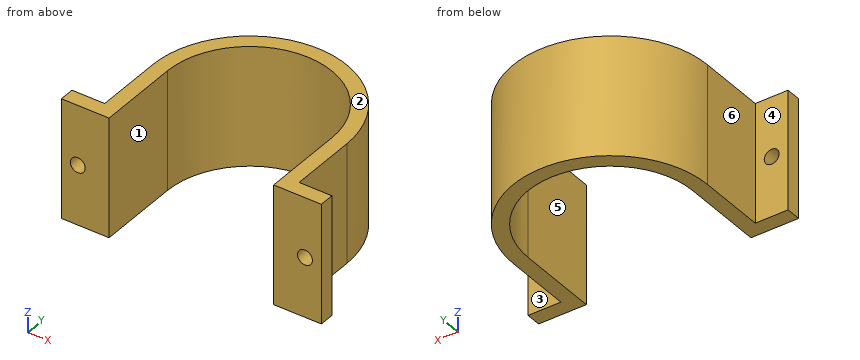
Autodesk Inventor part; units mm, degrees
ref_plane "YZ Plane" through (0, 0, 0) normal (1, 0, 0) x (0, 1, 0)
ref_plane "XZ Plane" through (0, 0, 0) normal (0, 1, 0) x (-1, 0, 0)
ref_plane "XY Plane" through (0, 0, 0) normal (0, 0, 1) x (1, 0, 0)
sketch "Sketch1" plane through (0, 0, 0) normal (0, 0, 1) x (1, 0, 0)
  arc A0 (17.526, 0) -> (-17.526, 0) centre (0, 0) ccw
  arc A1 (20.701, 0) -> (-20.701, 0) centre (0, 0) ccw
  line L0 (17.526, 0) -> (20.701, 0)
  line L1 (20.701, 0) -> (20.701, -17.526)
  line L2 (20.701, -17.526) -> (17.526, -17.526)
  line L3 (17.526, -17.526) -> (17.526, 0)
  line L4 (-20.701, 0) -> (-17.526, 0)
  line L5 (-17.526, 0) -> (-17.526, -17.526)
  line L6 (-17.526, -17.526) -> (-20.701, -17.526)
  line L7 (-20.701, -17.526) -> (-20.701, 0)
  line L8 (-17.526, -17.526) -> (-27.686, -17.526)
  line L9 (-27.686, -17.526) -> (-27.686, -14.351)
  line L10 (-27.686, -14.351) -> (-17.526, -14.351)
  line L11 (-17.526, -14.351) -> (-17.526, -17.526)
  line L12 (17.526, -17.526) -> (27.686, -17.526)
  line L13 (27.686, -17.526) -> (27.686, -14.351)
  line L14 (27.686, -14.351) -> (17.526, -14.351)
  line L15 (17.526, -14.351) -> (17.526, -17.526)
  point P0 (-20.701, -14.351)
  point P1 (20.701, -14.351)
  dimension "d0" = 17.526
  dimension "d1" = 3.175
  dimension "d23" = 3.175
  dimension "d24" = 17.526
  dimension "d25" = 3.175
  dimension "d26" = 17.526
  dimension "d27" = 10.16
  dimension "d28" = 3.175
  dimension "d29" = 10.16
  dimension "d30" = 3.175
extrude "Extrusion1" add sketch "Sketch1" along normal blind 25.4
sketch "Sketch5" plane through (-27.686, -14.351, 0) normal (0, 1, 0) x (1, 0, 0)
  line L0 (6.985, 0) -> (0, 0) construction
  line L1 (6.985, -25.4) -> (0, -25.4) construction
  line L2 (0, 0) -> (6.985, -25.4) construction
  line L3 (0, 0) -> (0, -25.4) construction
  line L4 (6.985, 0) -> (0, -25.4) construction
  line L5 (45.212, -25.4) -> (55.372, -25.4) construction
  line L6 (48.387, 0) -> (55.372, -25.4) construction
  line L7 (45.212, 0) -> (55.372, 0) construction
  line L8 (55.372, 0) -> (48.387, -25.4) construction
  point P0 (27.686, 0)
  point P1 (3.4925, -12.7)
sketch "Sketch6" plane through (20.701, -14.351, 0) normal (0, 1, 0) x (1, 0, 0)
  point P0 (-20.701, 0)
  point P1 (3.4926, -12.7006)
hole "Hole3" at (24.1936, -14.351, 12.7006) direction (0, -1, 0) diameter 3.175 end through all
hole "Hole4" at (-24.1935, -14.351, 12.7) direction (0, -1, 0) diameter 3.175 end through all
properties part number "ShootingMech_MotorMount"
Could you check a few things on this model? Use its own coordinates, in mm. Face numbers are marked on the shaded views. A direction names the side the tool comes from. Give positions to 0.01 mm unless a question says otherwise; leave off trailing zeros. Order: outer loops, then holes, each group sorted by start corner. A loop starts at its lowest first (then second) coordinate and runs counter-clockwise, first axis right, second up.
1. For pin 1 (3 mm diameter, centred on y = -12, z = 11, fed in from +X); pin 2 (3.5 mm diameter, centred on x = 25, z = 15.5, fed in from +Y); pin 3 (4 mm diameter, centred on x = -6, z = 5, fed in from +Y), each with a flat end and sliding along its axis, tell me the tip position at first contact or that it passes through.
Answers below:
pin 1: stops at x = 20.7
pin 2: stops at y = -14.35
pin 3: stops at y = 20.31
2. Which directions (+Z, -Z, +X, -X, +Y, -Y) give clear straight access to the entire face, cutting with the end or side of a thin tool? Please do the marked faces 1, 2 and 3.
Answers below:
face 1: +Z, -Z, -Y
face 2: +Z, +X, -X, +Y, -Y
face 3: +Z, -Z, +X, +Y
3. I need wall thicknesses on L1, parallel to X at y = -5, z = 3.5; L2, parallel to X at y = -15.7, z = 12.7; L3, parallel to X at y = 12, z = 6.5. Which ranges of each line are inside material? Lowest first, please.
Answers below:
L1: x = -20.7 to -17.53, 17.53 to 20.7
L2: x = -27.69 to -25.78, -22.61 to -17.53, 17.53 to 22.61, 25.78 to 27.69
L3: x = -16.87 to -12.77, 12.77 to 16.87
4. Suppose I cut it at B-B (y = -15). Write out the boundary of the cut face in (x, z) (1 decimal).
Answers below:
outline: (-27.7, 0) - (-17.5, 0) - (-17.5, 25.4) - (-27.7, 25.4) - close; (17.5, 0) - (27.7, 0) - (27.7, 25.4) - (17.5, 25.4) - close; hole circle Ø3.2 at (-24.2, 12.7); hole circle Ø3.2 at (24.2, 12.7)
5. Thinking about a two-plate mould opening in X: for the marked faces 4, 5 and 6, which applies, +X half, -X half, draft (parallel to the pull), parting line (faces both ways), or undercut?
Answers below:
face 4: draft
face 5: undercut
face 6: -X half
6. Suppose I cut it at D-D (x = 0). Write out the boundary of the cut face in (y, z).
Answers below:
outline: (17.53, 0) - (20.7, 0) - (20.7, 25.4) - (17.53, 25.4) - close
7. Suppose I cut it at A-A (y = -8). Write out the boundary of the cut face in (x, z).
Answers below:
outline: (-20.7, 0) - (-17.53, 0) - (-17.53, 25.4) - (-20.7, 25.4) - close; (17.53, 0) - (20.7, 0) - (20.7, 25.4) - (17.53, 25.4) - close
8. Suppose I cut it at C-C (z = 12.7). Write out the boundary of the cut face in (x, y), plus the area to 3 significant figures.
Answers below:
outline: (-27.69, -17.53) - (-25.78, -17.53) - (-25.78, -14.35) - (-27.69, -14.35) - close; (-22.61, -17.53) - (-17.53, -17.53) - (-17.53, 0) arc R17.53 cw to (17.53, 0) - (17.53, -17.53) - (22.61, -17.53) - (22.61, -14.35) - (20.7, -14.35) - (20.7, 0) arc R20.7 ccw to (-20.7, 0) - (-20.7, -14.35) - (-22.61, -14.35) - close; (25.78, -17.53) - (27.69, -17.53) - (27.69, -14.35) - (25.78, -14.35) - close
area: 326 mm2
